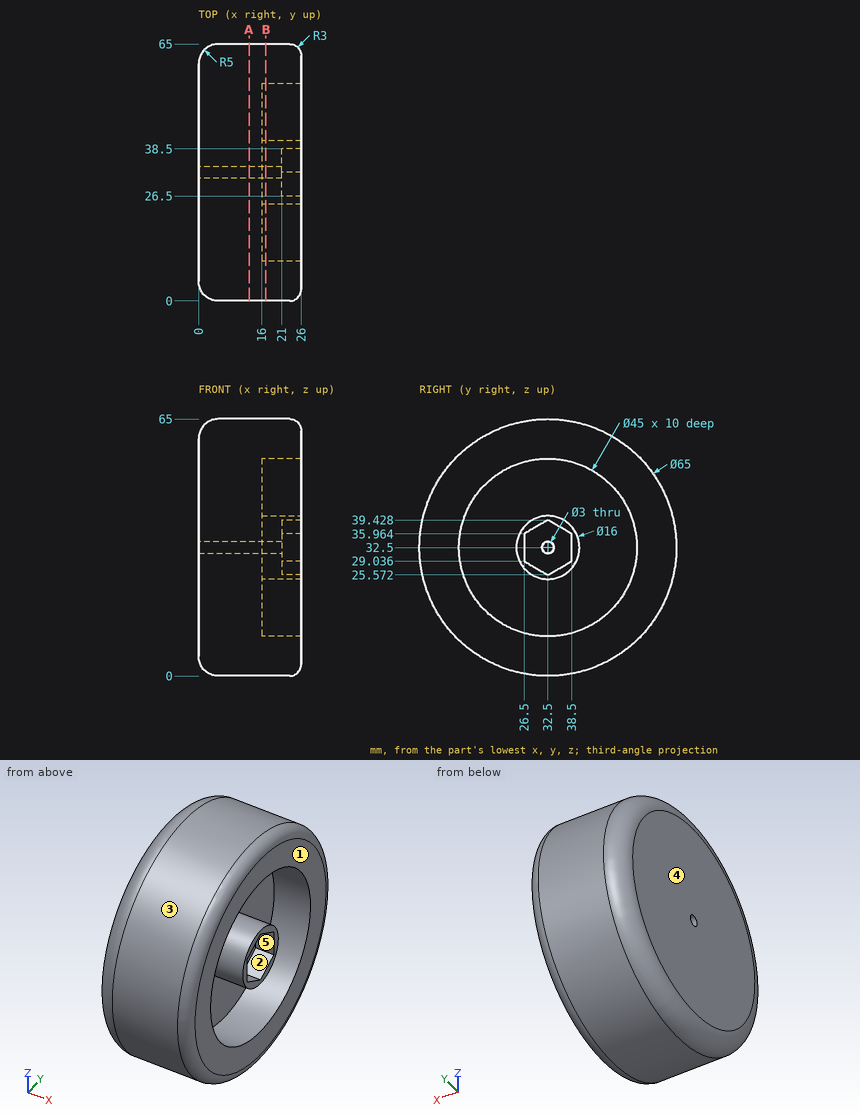
Could you check a few things on this drawing? It's one solid part, dimensions in mm from its lowest x, y, z. A direction names the side the tool comes from. Coordinates: 2 decimals unless noted, no trailing zeros. Write each loop counter-clockwise with the first axis right and the second up, starting at its lowest first coordinate (ties: lowest second). Pieces come first, ordered by that corner, then holes. Notation, with made-up numbers: (17, 43) - (30, 43) arc R29 cw to (30, 75) - close; hole circle Ø9 at (42, 74). An arc over 180 degrees is marked (long way). Write item = value, one per line.
1) Suppose I cut it at B-B on x = 17. Please give me the cut outline in (y, z), plus the area to 3 significant figures.
Result set:
outline = circle Ø65 at (32.5, 32.5); circle Ø16 at (32.5, 32.5); hole circle Ø45 at (32.5, 32.5); hole circle Ø3 at (32.5, 32.5)
area = 1,920 mm2
2) We'd pull the mould along Y, two halves only. Please class the marked faces 1, 2 and 3: +Y half, -Y half, draft (parallel to the pull), parting line (faces both ways), or undercut.
Result set:
face_1 = draft
face_2 = undercut
face_3 = parting line
3) Please list where these lines run through material, in increasing order: line 1 (Y direction, x = 19.25, z = 32.5); line 2 (Y direction, x = 6.5, z = 32.5); line 3 (Y direction, x = 19, z = 32) (1 decimal). Write a range as [from, to].
Result set:
line_1 = [0, 10], [24.5, 31], [34, 40.5], [55, 65]
line_2 = [0, 31], [34, 65]
line_3 = [0, 10], [24.5, 31.1], [33.9, 40.5], [55, 65]
4) For the marked faces 4 and 5, which set-ups out of +Z, -Z, +X, -X, +Y, -Y let a thin tool reach every point of the face, with its end or its side?
Result set:
face_4 = +Z, -Z, -X, +Y, -Y
face_5 = +X
5) Suppose I cut it at A-A on x = 12.75. Please give me the cut outline in (y, z).
Result set:
outline = circle Ø65 at (32.5, 32.5); hole circle Ø3 at (32.5, 32.5)
6) Will these pins go through, and if not, where does the flat tip stop? pin 1 Ø3 at (x, y) = (12, 55.5) entering from +Z; pin 2 Ø8 at (x, y) = (10.5, 23.5) entering from +Z; pin 3 Ø4 at (x, z) = (21, 35) entering from -Y.
Result set:
pin_1 = 56.87
pin_2 = 64.61
pin_3 = 0
